Geometry: final body of the model. Coordinates: model frame, mm. A direction names the side the tool comes from. Give positions to 0.01 mm unless a question says otherwise; leave off trailing zeros. One line per question, with ' | ' between items.
from build123d import *

# Parameters (mm, degrees)
BOSS_EXTRUDE1_DEPTH = 280


with BuildPart() as part:
    # Sketch1 → Boss-Extrude1 (new body)
    with BuildSketch(Plane.XY.offset(4000)):
        with BuildLine():
            Line((10, 3.138), (10, 8.5))
            ThreePointArc((10, 8.5), (9.560660172, 9.560660172), (8.5, 10))
            Line((8.5, 10), (3.138, 10))
            ThreePointArc((3.138, 10), (2.778789755, 9.851210245), (2.63, 9.492))
            Line((2.63, 9.492), (2.63, 9.008))
            ThreePointArc((2.63, 9.008), (2.778789755, 8.648789755), (3.138, 8.5))
            Line((3.138, 8.5), (5.487, 8.5))
            ThreePointArc((5.487, 8.5), (5.846210245, 8.351210245), (5.995, 7.992))
            Line((5.995, 7.992), (5.995, 7.266080661))
            ThreePointArc((5.995, 7.266080661), (5.956330803, 7.071677478), (5.846210245, 6.906870417))
            Line((5.846210245, 6.906870417), (2.743129583, 3.803789755))
            ThreePointArc((2.743129583, 3.803789755), (2.578322522, 3.693669197), (2.383919339, 3.655))
            Line((2.383919339, 3.655), (-2.383919339, 3.655))
            ThreePointArc((-2.383919339, 3.655), (-2.578322522, 3.693669197), (-2.743129583, 3.803789755))
            Line((-2.743129583, 3.803789755), (-5.846210245, 6.906870417))
            ThreePointArc((-5.846210245, 6.906870417), (-5.956330803, 7.071677478), (-5.995, 7.266080661))
            Line((-5.995, 7.266080661), (-5.995, 7.992))
            ThreePointArc((-5.995, 7.992), (-5.846210245, 8.351210245), (-5.487, 8.5))
            Line((-5.487, 8.5), (-3.138, 8.5))
            ThreePointArc((-3.138, 8.5), (-2.778789755, 8.648789755), (-2.63, 9.008))
            Line((-2.63, 9.008), (-2.63, 9.492))
            ThreePointArc((-2.63, 9.492), (-2.778789755, 9.851210245), (-3.138, 10))
            Line((-3.138, 10), (-8.5, 10))
            ThreePointArc((-8.5, 10), (-9.560660172, 9.560660172), (-10, 8.5))
            Line((-10, 8.5), (-10, 3.138))
            ThreePointArc((-10, 3.138), (-9.851210245, 2.778789755), (-9.492, 2.63))
            Line((-9.492, 2.63), (-9.008, 2.63))
            ThreePointArc((-9.008, 2.63), (-8.648789755, 2.778789755), (-8.5, 3.138))
            Line((-8.5, 3.138), (-8.5, 5.487))
            ThreePointArc((-8.5, 5.487), (-8.351210245, 5.846210245), (-7.992, 5.995))
            Line((-7.992, 5.995), (-7.266080661, 5.995))
            ThreePointArc((-7.266080661, 5.995), (-7.071677478, 5.956330803), (-6.906870417, 5.846210245))
            Line((-6.906870417, 5.846210245), (-3.803789755, 2.743129583))
            ThreePointArc((-3.803789755, 2.743129583), (-3.693669197, 2.578322522), (-3.655, 2.383919339))
            Line((-3.655, 2.383919339), (-3.655, -2.383919339))
            ThreePointArc((-3.655, -2.383919339), (-3.693669197, -2.578322522), (-3.803789755, -2.743129583))
            Line((-3.803789755, -2.743129583), (-6.906870417, -5.846210245))
            ThreePointArc((-6.906870417, -5.846210245), (-7.071677478, -5.956330803), (-7.266080661, -5.995))
            Line((-7.266080661, -5.995), (-7.992, -5.995))
            ThreePointArc((-7.992, -5.995), (-8.351210245, -5.846210245), (-8.5, -5.487))
            Line((-8.5, -5.487), (-8.5, -3.138))
            ThreePointArc((-8.5, -3.138), (-8.648789755, -2.778789755), (-9.008, -2.63))
            Line((-9.008, -2.63), (-9.492, -2.63))
            ThreePointArc((-9.492, -2.63), (-9.851210245, -2.778789755), (-10, -3.138))
            Line((-10, -3.138), (-10, -8.5))
            ThreePointArc((-10, -8.5), (-9.560660172, -9.560660172), (-8.5, -10))
            Line((-8.5, -10), (-3.138, -10))
            ThreePointArc((-3.138, -10), (-2.778789755, -9.851210245), (-2.63, -9.492))
            Line((-2.63, -9.492), (-2.63, -9.008))
            ThreePointArc((-2.63, -9.008), (-2.778789755, -8.648789755), (-3.138, -8.5))
            Line((-3.138, -8.5), (-5.487, -8.5))
            ThreePointArc((-5.487, -8.5), (-5.846210245, -8.351210245), (-5.995, -7.992))
            Line((-5.995, -7.992), (-5.995, -7.266080661))
            ThreePointArc((-5.995, -7.266080661), (-5.956330803, -7.071677478), (-5.846210245, -6.906870417))
            Line((-5.846210245, -6.906870417), (-2.743129583, -3.803789755))
            ThreePointArc((-2.743129583, -3.803789755), (-2.578322522, -3.693669197), (-2.383919339, -3.655))
            Line((-2.383919339, -3.655), (2.383919339, -3.655))
            ThreePointArc((2.383919339, -3.655), (2.578322522, -3.693669197), (2.743129583, -3.803789755))
            Line((2.743129583, -3.803789755), (5.846210245, -6.906870417))
            ThreePointArc((5.846210245, -6.906870417), (5.956330803, -7.071677478), (5.995, -7.266080661))
            Line((5.995, -7.266080661), (5.995, -7.992))
            ThreePointArc((5.995, -7.992), (5.846210245, -8.351210245), (5.487, -8.5))
            Line((5.487, -8.5), (3.138, -8.5))
            ThreePointArc((3.138, -8.5), (2.778789755, -8.648789755), (2.63, -9.008))
            Line((2.63, -9.008), (2.63, -9.492))
            ThreePointArc((2.63, -9.492), (2.778789755, -9.851210245), (3.138, -10))
            Line((3.138, -10), (8.5, -10))
            ThreePointArc((8.5, -10), (9.560660172, -9.560660172), (10, -8.5))
            Line((10, -8.5), (10, -3.138))
            ThreePointArc((10, -3.138), (9.851210245, -2.778789755), (9.492, -2.63))
            Line((9.492, -2.63), (9.008, -2.63))
            ThreePointArc((9.008, -2.63), (8.648789755, -2.778789755), (8.5, -3.138))
            Line((8.5, -3.138), (8.5, -5.487))
            ThreePointArc((8.5, -5.487), (8.351210245, -5.846210245), (7.992, -5.995))
            Line((7.992, -5.995), (7.266080661, -5.995))
            ThreePointArc((7.266080661, -5.995), (7.071677478, -5.956330803), (6.906870417, -5.846210245))
            Line((6.906870417, -5.846210245), (3.803789755, -2.743129583))
            ThreePointArc((3.803789755, -2.743129583), (3.693669197, -2.578322522), (3.655, -2.383919339))
            Line((3.655, -2.383919339), (3.655, 2.383919339))
            ThreePointArc((3.655, 2.383919339), (3.693669197, 2.578322522), (3.803789755, 2.743129583))
            Line((3.803789755, 2.743129583), (6.906870417, 5.846210245))
            ThreePointArc((6.906870417, 5.846210245), (7.071677478, 5.956330803), (7.266080661, 5.995))
            Line((7.266080661, 5.995), (7.992, 5.995))
            ThreePointArc((7.992, 5.995), (8.351210245, 5.846210245), (8.5, 5.487))
            Line((8.5, 5.487), (8.5, 3.138))
            ThreePointArc((8.5, 3.138), (8.648789755, 2.778789755), (9.008, 2.63))
            Line((9.008, 2.63), (9.492, 2.63))
            ThreePointArc((9.492, 2.63), (9.851210245, 2.778789755), (10, 3.138))
        make_face()
        with BuildLine():
            Line((-2.124900844, -2.304505966), (-2.304505966, -2.124900844))
            ThreePointArc((-2.304505966, -2.124900844), (-2.505938017, -1.356467811), (-1.935133506, -0.803976718))
            ThreePointArc((-1.935133506, -0.803976718), (-2.0955, 0), (-1.935133506, 0.803976718))
            ThreePointArc((-1.935133506, 0.803976718), (-2.505938017, 1.356467811), (-2.304505966, 2.124900844))
            Line((-2.304505966, 2.124900844), (-2.124900844, 2.304505966))
            ThreePointArc((-2.124900844, 2.304505966), (-1.356467811, 2.505938017), (-0.803976718, 1.935133506))
            ThreePointArc((-0.803976718, 1.935133506), (0, 2.0955), (0.803976718, 1.935133506))
            ThreePointArc((0.803976718, 1.935133506), (1.356467811, 2.505938017), (2.124900844, 2.304505966))
            Line((2.124900844, 2.304505966), (2.304505966, 2.124900844))
            ThreePointArc((2.304505966, 2.124900844), (2.505938017, 1.356467811), (1.935133506, 0.803976718))
            ThreePointArc((1.935133506, 0.803976718), (2.0955, 0), (1.935133506, -0.803976718))
            ThreePointArc((1.935133506, -0.803976718), (2.505938017, -1.356467811), (2.304505966, -2.124900844))
            Line((2.304505966, -2.124900844), (2.124900844, -2.304505966))
            ThreePointArc((2.124900844, -2.304505966), (1.356467811, -2.505938017), (0.803976718, -1.935133506))
            ThreePointArc((0.803976718, -1.935133506), (0, -2.0955), (-0.803976718, -1.935133506))
            ThreePointArc((-0.803976718, -1.935133506), (-1.356467811, -2.505938017), (-2.124900844, -2.304505966))
        make_face(mode=Mode.SUBTRACT)
    extrude(amount=-BOSS_EXTRUDE1_DEPTH)


solid = part.part
1) Material intervals for probe 1 along X at (y, z) = (-8, 3864.5); probe 2 along X at (y, z) = (-4.25, 3911); probe 3 along X at (y, z) = (-4, 3814), sorted ascending. Write a range as from..to.
Check result:
probe 1: x = -10..-5.99, 5.99..10 | probe 2: x = -10..-8.5, -5.31..-3.19, 3.19..5.31, 8.5..10 | probe 3: x = -10..-8.5, -5.06..-2.94, 2.94..5.06, 8.5..10
2) Contact query for flat-ended pins moving along their axis: pin 1 Ø3 at (x, z) = (0.5, 3850.5) entering from +Y (3 decimals); pin 2 Ø4 at (y, z) = (-1, 3910.5) entering from -X; pin 3 Ø1.4 at (x, z) = (0, 3806.5) entering from -Y (3 decimals). Output: stop coordinate, or through.
Check result:
pin 1: stops at y = 3.655 | pin 2: stops at x = -9.98 | pin 3: stops at y = -3.655
3) Pull-direction query (X, two-part tool) for faces 6 (the flat face through (10, 6, 3862)), 7 (the flat face through (-6, -10, 3862)), 8 (the flat face through (0, 3.655, 3862)); classes: +X half, -X half, draft (parallel to the pull), parting line (faces both ways), or undercut.
Check result:
face 6: +X half | face 7: draft | face 8: undercut
4) Set-up query: faces 1 (the flat face through (6, 10, 3862)), 2 (the flat face through (0, -3.655, 3862)), 3 (the flat face through (-3.655, 0, 3862)), 4 (the flat face through (10, -6, 3862)), 5 (the flat face through (3.655, 0, 3862)). Return all of +Z, -Z, +X, -X, +Y, -Y with unobstructed straight access to the full face (end or side cutting, diameter ignored); none if empty.
Check result:
face 1: +Z, -Z, +X, -X, +Y | face 2: +Z, -Z, -Y | face 3: +Z, -Z, -X | face 4: +Z, -Z, +X, +Y, -Y | face 5: +Z, -Z, +X
